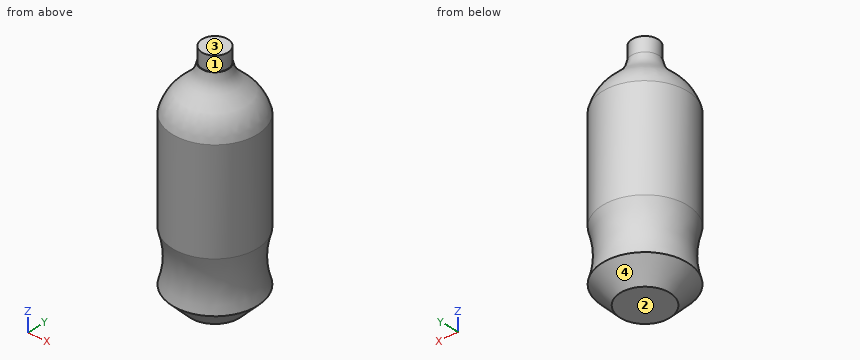
```python
from build123d import *


with BuildPart() as f1:
    # F0 (on Right) → F1 (revolve)
    with BuildSketch(Plane.YZ):
        with BuildLine():
            Line((0, -31.489287), (0, -32.924928))
            Line((0, -32.924928), (11.622462, -32.924928))
            Line((11.622462, -32.924928), (19.999593, -24.056212))
            add(Edge.make_bspline(
                [(19.999593, -24.056212), (17.396746, -16.114077), (17.657735, -7.724358), (19.999593, 0)],
                knots=[0, 0, 0, 0, 24.056212, 24.056212, 24.056212, 24.056212], degree=3))
            Line((19.999593, 0), (19.999593, 47.861013))
            add(Edge.make_bspline(
                [(19.999593, 47.861013), (16.597867, 60.171429), (7.622306, 59.965661), (6.374207, 69.110181)],
                knots=[0, 0, 0, 0, 25.24239, 25.24239, 25.24239, 25.24239], degree=3))
            Line((6.374207, 69.110181), (6.358525, 69.110181))
            Line((6.358525, 69.110181), (6.111381, 69.110181))
            Line((6.111381, 69.110181), (5.864237, 69.110181))
            add(Edge.make_bspline(
                [(5.864237, 69.110181), (6.431991, 59.965661), (16.597867, 58.923964), (18.760797, 48.862453)],
                knots=[0, 0, 0, 0, 24.006077, 24.006077, 24.006077, 24.006077], degree=3))
            Line((18.760797, 48.862453), (18.760797, 0))
            add(Edge.make_bspline(
                [(18.760797, 0), (16.353968, -7.724358), (17.396746, -16.114077), (18.760797, -24.074806)],
                knots=[0, 0, 0, 0, 24.074806, 24.074806, 24.074806, 24.074806], degree=3))
            Line((18.760797, -24.074806), (11.757294, -31.489287))
            Line((11.757294, -31.489287), (0, -31.489287))
        make_face()
        Polygon((0, 75.95484), (0, 69.110181), (5.864237, 69.110181), (6.111381, 69.110181), (6.111381, 75.95484), align=None)
    revolve(axis=Axis((0, 0, 10.99069), (0, 0, 1)))


solid = f1.part
```
Verification items for the finished model (mm, model axes). Face numbers are marked on the shaded views. A direction names the side the tool comes from. Give positions to 0.01 mm unless a question says otherwise; leave off trailing zeros. Order: outer loops, then holes, each group sorted by start corner. A loop starts at its lowest first (then second) coordinate and runs counter-clockwise, first axis right, second up. Notation, with made-up numbers: (-17, 28) -> (38, 28) arc R14 cw to (38, 39) -> close; hole circle Ø8 at (-6, -38). An arc over 180 degrees is marked (long way). Use a Markdown table: item, result.
1) Depth check by flat-ended pin: pin 1 Ø19 at (x, y) = (-5, -4) entering from +Z; pin 2 Ø1 at (y, z) = (1.5, 4) entering from -X; pin 3 Ø5 at (y, z) = (-1, 57) entering from -X; pin 4 Ø2 at (x, y) = (-11, -10.5) entering from +Z. Enter the tip coordinate at first touch or a pass-through.
Results:
| item | result |
|---|---|
| pin 1 | z = 75.95 |
| pin 2 | x = -19.97 |
| pin 3 | x = -17 |
| pin 4 | z = 57.91 |
2) Section check A-A, the plane z = 10. Record the boundary of the cut face in (x, y).
Results:
| item | result |
|---|---|
| outline | circle Ø40 at (0, 0); hole circle Ø37.52 at (0, 0) |
3) Mould release check, pull along X, two halves, no side actions. Record for the marked faces 3 and 4: pulls with the +X half, pulls with the -X half, needs draft (parallel to the pull), parting line crosses it, or undercut.
Results:
| item | result |
|---|---|
| face 3 | needs draft |
| face 4 | parting line crosses it |
4) Material ranges on probe 1 along X at (y, z) = (0, 33.5); probe 2 along X at (y, z) = (-10, 49.5), recorded low to high.
Results:
| item | result |
|---|---|
| probe 1 | -20 to -18.76, 18.76 to 20 |
| probe 2 | -16.73 to -15.7, 15.7 to 16.73 |
5) Tool access check on the marked faces 1 and 2. Record the directions out of +Z, -Z, +X, -X, +Y, -Y that give a thin tool (end or side, any length) a straight path to the whole face; none if there is none.
Results:
| item | result |
|---|---|
| face 1 | +Z |
| face 2 | -Z, +X, -X, +Y, -Y |
